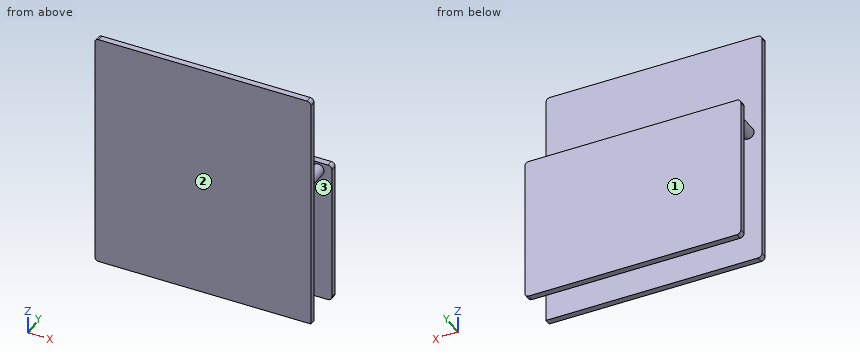
from build123d import *

# Parameters (mm, degrees)
SKETCH1_W           = 55
SKETCH1_H           = 61
BOSS_EXTRUDE1_DEPTH = 1.6
SKETCH2_R           = 1.5
BOSS_EXTRUDE2_DEPTH = 8.8
SKETCH3_W           = 55
SKETCH3_H           = 37
BOSS_EXTRUDE3_DEPTH = 1.6
FILLET1_R           = 1


with BuildPart() as part:
    # Sketch1 → Boss-Extrude1 (new body)
    with BuildSketch(Plane(origin=(0, 0, 0), x_dir=(1, 0, 0), z_dir=(0, 1, 0))):
        Rectangle(SKETCH1_W, SKETCH1_H)
    extrude(amount=BOSS_EXTRUDE1_DEPTH)

    # Sketch2 → Boss-Extrude2 (add)
    with BuildSketch(Plane(origin=(0, 1.6, 0), x_dir=(1, 0, 0), z_dir=(0, 1, 0))):
        with Locations(Location((-24, -4.5, 0), (0, 0, 270))):
            Circle(SKETCH2_R)
        with Locations(Location((24, -4.5, 0), (0, 0, 270))):
            Circle(SKETCH2_R)
    extrude(amount=BOSS_EXTRUDE2_DEPTH)

    # Sketch3 → Boss-Extrude3 (add)
    with BuildSketch(Plane(origin=(0, 10.4, 0), x_dir=(1, 0, 0), z_dir=(0, 1, 0))):
        with Locations((0, 12)):
            Rectangle(SKETCH3_W, SKETCH3_H)
    extrude(amount=BOSS_EXTRUDE3_DEPTH)

    # Fillet1
    fillet1_edges = [part.edges().sort_by_distance(p)[0] for p in [
        (-27.5, 11.2, -30.5),
        (-27.5, 11.2, 6.5),
        (27.5, 11.2, 6.5),
        (27.5, 11.2, -30.5),
        (-27.5, 0.8, -30.5),
        (27.5, 0.8, 30.5),
        (-27.5, 0.8, 30.5),
    ]]
    fillet(fillet1_edges, radius=FILLET1_R)


solid = part.part
The listing builds one solid part. Answer for the finished solid, in the listing's coordinates (mm). Face numbers are marked on the shaded views. Coordinates: 2 decimals unless noted, no trailing zeros. Order: outer loops, then holes, each group sorted by start corner. A loop starts at its lowest first (then second) coordinate and runs counter-clockwise, first axis right, second up. Notation, with made-up numbers: (87, 61) -> (124, 61) arc R8 ccw to (124, 75) -> close; hole circle Ø3 at (-32.75, -24). An arc over 180 degrees is marked (long way). Answer in a Markdown table with one row per item. Add a question column.
Item 1: Each of these flat-tipped pins is pushed along its axis until it touches: P1, Ø1.5, axis at y = 9, z = 2.5, coming from the +X side; P2, Ø1, axis at x = 21, z = -21, coming from the -Y side; P3, Ø1.5, axis at y = 4, z = 1, coming from the +X side; P4, Ø1.3, axis at x = -0.5, y = 11.5, coming from the +Z side. Where does it stop, or does it pass through?
Item 2: Determine the mould class of the marked faces 1, 2 and 3 for opening direction Y: +Y half, -Y half, draft (parallel to the pull), parting line (faces both ways), or undercut.
Item 3: Find section B-B (x = -1). Write down the section's boundary in (y, z).
Item 4: Find section A-A (z = -23). Write down the section's boundary in (x, y), then the cut area to 3 significant figures.
Item 5: Find section C-C (y = 7). Write down the section's boundary in (x, z).
Item 6: Find section D-D (x = 24). Write down the section's boundary in (y, z).
Item 7: Find the intervals of material crossed by L1, parallel to Y at x = 25.5, z = -3; L2, parallel to Y at x = 22.5, z = 16.5; L3, parallel to Z at x = 25.5, y = 11.25, in increasing order. Write a range as from..to.
Result set:
| question | item | result |
|---|---|---|
| 1 | P1 | stops at x = 24.83 |
| 1 | P2 | stops at y = 0 |
| 1 | P3 | passes through |
| 1 | P4 | stops at z = 6.5 |
| 2 | face 1 | +Y half |
| 2 | face 2 | -Y half |
| 2 | face 3 | undercut |
| 3 | outline | (0, -30.5) -> (1.6, -30.5) -> (1.6, 30.5) -> (0, 30.5) -> close; (10.4, -30.5) -> (12, -30.5) -> (12, 6.5) -> (10.4, 6.5) -> close |
| 4 | outline | (-27.5, 0) -> (27.5, 0) -> (27.5, 1.6) -> (-27.5, 1.6) -> close; (-27.5, 10.4) -> (27.5, 10.4) -> (27.5, 12) -> (-27.5, 12) -> close |
| 4 | area | 176 mm² |
| 5 | outline | circle Ø3 at (-24, 4.5); circle Ø3 at (24, 4.5) |
| 6 | outline | (0, -30.5) -> (1.6, -30.5) -> (1.6, 3) -> (10.4, 3) -> (10.4, -30.5) -> (12, -30.5) -> (12, 6.5) -> (10.4, 6.5) -> (10.4, 6) -> (1.6, 6) -> (1.6, 30.5) -> (0, 30.5) -> close |
| 7 | L1 | y = 0..1.6, 10.4..12 |
| 7 | L2 | y = 0..1.6 |
| 7 | L3 | z = -30.5..6.5 |
